```python
from build123d import *

# Parameters (mm, degrees)
F0_W          = 134.0631097555
F0_H          = 82.4345424771
F1_DEPTH      = 38.1
F1_DEPTH_BACK = 38.1
F2_R          = 11.3246281271
F3_DEPTH      = 93.726
F3_DEPTH_BACK = 71.374
F4_W          = 68.1725181639
F4_H          = 33.9436363429
F5_DEPTH      = 44.958
F5_DEPTH_BACK = 59.69
F6_W          = 122.6534843445
F6_H          = 65.8905878663
F7_DEPTH      = 79.756
F7_DEPTH_BACK = 65.786


with BuildPart() as f1:
    # F0 (on Front) → F1 (new body, two sides)
    with BuildSketch(Plane.XZ) as f1_sk:
        Rectangle(F0_W, F0_H)
    extrude(amount=F1_DEPTH)
    extrude(f1_sk.sketch, amount=-F1_DEPTH_BACK)

    # F2 (on Right) → F3 (cut, two sides)
    with BuildSketch(Plane.YZ) as f3_sk:
        Circle(F2_R)
    extrude(amount=F3_DEPTH, mode=Mode.SUBTRACT)
    extrude(f3_sk.sketch, amount=-F3_DEPTH_BACK, mode=Mode.SUBTRACT)

    # F4 (on Front) → F5 (cut, two sides)
    with BuildSketch(Plane.XZ) as f5_sk:
        with Locations((1.2835841626, 39.9336898699)):
            Rectangle(F4_W, F4_H)
    extrude(amount=-F5_DEPTH, mode=Mode.SUBTRACT)
    extrude(f5_sk.sketch, amount=F5_DEPTH_BACK, mode=Mode.SUBTRACT)

    # F6 (on Top) → F7 (cut, two sides)
    with BuildSketch(Plane.XY) as f7_sk:
        Rectangle(F6_W, F6_H)
    extrude(amount=-F7_DEPTH, mode=Mode.SUBTRACT)
    extrude(f7_sk.sketch, amount=F7_DEPTH_BACK, mode=Mode.SUBTRACT)


solid = f1.part
```
Geometry check sheet. Reference: the model listing, model coordinates, mm. A direction names the side the tool comes from. Give positions to 0.01 mm unless a question says otherwise; leave off trailing zeros. Loops run counter-clockwise (first coordinate to the right, second up) from the corner with the lowest first, then second, coordinate; pieces in that order, holes last. Notation, with made-up numbers: M 39.25,3.25 L 44.25,3.25 A5 ccw 44.25,9.25 Z; hole C 48,-30 d8. An arc over 180 degrees is marked long. Write item = value, one per line.
(1) Material ranges on line 1 (X direction, y = 14, z = -2); line 2 (Z direction, x = 63, y = 0); line 3 (Y direction, x = 42, z = 4), recorded low to high. Write a range as [from, to].
Answer below:
line_1 = [-67.03, -61.33], [61.33, 67.03]
line_2 = [-41.22, -11.32], [11.32, 41.22]
line_3 = [-38.1, -32.95], [32.95, 38.1]
(2) Sectioned sample at D-D, the plane x = 53.5. Record the cut outline in (y, z).
Answer below:
outline = M -38.1,-41.22 L -32.95,-41.22 L -32.95,41.22 L -38.1,41.22 Z; M 32.95,-41.22 L 38.1,-41.22 L 38.1,41.22 L 32.95,41.22 Z
(3) Sectioned sample at B-B, the plane z = 0. Record the cut outline in (x, y), plus the area to 3 significant figures.
Answer below:
outline = M -67.03,-38.1 L 67.03,-38.1 L 67.03,-11.32 L 61.33,-11.32 L 61.33,-32.95 L -61.33,-32.95 L -61.33,-11.32 L -67.03,-11.32 Z; M -67.03,11.32 L -61.33,11.32 L -61.33,32.95 L 61.33,32.95 L 61.33,11.32 L 67.03,11.32 L 67.03,38.1 L -67.03,38.1 Z
area = 1,880 mm2
(4) Gauge pin test, flat ends, axial feed: pin 1 Ø20 at (y, z) = (2.5, -8) entering from +X; pin 2 Ø4 at (x, y) = (2, -35.5) entering from +Z; pin 3 Ø18 at (y, z) = (0, 0) entering from +X. Record the tip position at first contact, or that the pin passes through.
Answer below:
pin_1 = 67.03
pin_2 = 22.96
pin_3 = through
(5) Sectioned sample at C-C, the plane x = -21. Record the cut outline in (y, z), plus the area to 3 significant figures.
Answer below:
outline = M -38.1,-41.22 L -32.95,-41.22 L -32.95,22.96 L -38.1,22.96 Z; M 32.95,-41.22 L 38.1,-41.22 L 38.1,22.96 L 32.95,22.96 Z
area = 662 mm2
(6) Sectioned sample at A-A, the plane y = 0. Record the cut outline in (x, z).
Answer below:
outline = M -67.03,-41.22 L -61.33,-41.22 L -61.33,-11.32 L -67.03,-11.32 Z; M -67.03,11.32 L -61.33,11.32 L -61.33,41.22 L -67.03,41.22 Z; M 61.33,-41.22 L 67.03,-41.22 L 67.03,-11.32 L 61.33,-11.32 Z; M 61.33,11.32 L 67.03,11.32 L 67.03,41.22 L 61.33,41.22 Z
(7) Release check for a two-part mould opening along Y. For faces 1 (the face through (-1, 32.945, 1)), 2 (the face through (61.327, -8, 10)), 3 (the face through (35.37, 35, 32)), 4 (the face through (-1, -38.1, 1)) record: released by +Y, released by -Y, zero draft, split by the parting line, or undercut.
Answer below:
face_1 = undercut
face_2 = undercut
face_3 = zero draft
face_4 = released by -Y
(8) Tool access check on faces 5 (the face through (-32.803, 35, 32)), 6 (the face through (-62, -1, 41.217)), 7 (the face through (-1, -32.945, 1)). Record the directions out of +Z, -Z, +X, -X, +Y, -Y that give a thin tool (end or side, any length) a straight path to the whole face; none if there is none.
Answer below:
face_5 = +Z, +Y, -Y
face_6 = +Z, +X, -X, +Y, -Y
face_7 = +Z, -Z
